Source: CAD feature listing. Evaluate the final solid. Frame: model axes, mm. Give positions to 0.01 mm unless a question says otherwise; leave off trailing zeros. Loops run counter-clockwise (first coordinate to the right, second up) from the corner with the lowest first, then second, coordinate; pieces in that order, holes last. Notation, with made-up numbers: M 26,-5.5 L 72,-5.5 A22 ccw 72,9.5 Z; hole C 26.5,42.5 d6. An arc over 180 degrees is marked long. Write item = value, one per line.
from build123d import *

# Parameters (mm, degrees)
F0_R     = 18.669
F1_DEPTH = 3.302


# Not quite as in the source:
# - a length typed as a fraction of an inch, garbled in the dataset ("3 / 203.2 mm" for 3/8 in), is restored


with BuildPart() as f1:
    # F0 (on Top) → F1 (new body)
    with BuildSketch(Plane.XY):
        Circle(F0_R)
        Polygon((-5.6092465283, 3.2385000208), (-3.7394976935, 6.477), (0, 6.477), (3.7394976935, 6.477), (5.6092465069, 3.238500058), (7.4789953871, 0), (5.6092465631, -3.2384999606), (3.7394976935, -6.477), (0, -6.477), (-3.7394976935, -6.477), (-5.6092464752, -3.2385001127), (-7.4789953871, 0), align=None, mode=Mode.SUBTRACT)
        with BuildLine():
            Line((0, 6.477), (-3.7394976935, 6.477))
            Line((-3.7394976935, 6.477), (-5.6092465283, 3.2385000208))
            ThreePointArc((-5.6092465283, 3.2385000208), (-3.2384999896, 5.6092465463), (0, 6.477))
        make_face()
        with BuildLine():
            Line((3.7394976935, 6.477), (0, 6.477))
            ThreePointArc((0, 6.477), (3.238499971, 5.609246557), (5.6092465069, 3.238500058))
            Line((5.6092465069, 3.238500058), (3.7394976935, 6.477))
        make_face()
        with BuildLine():
            ThreePointArc((5.6092465631, -3.2384999606), (3.2385000197, -5.6092465289), (0, -6.477))
            Line((0, -6.477), (3.7394976935, -6.477))
            Line((3.7394976935, -6.477), (5.6092465631, -3.2384999606))
        make_face()
        with BuildLine():
            Line((7.4789953871, 0), (5.6092465069, 3.238500058))
            ThreePointArc((5.6092465069, 3.238500058), (6.2563015682, 1.6763709874), (6.477, 0))
            ThreePointArc((6.477, 0), (6.2563015828, -1.6763709332), (5.6092465631, -3.2384999606))
            Line((5.6092465631, -3.2384999606), (7.4789953871, 0))
        make_face()
        with BuildLine():
            ThreePointArc((0, -6.477), (-3.2384999437, -5.6092465728), (-5.6092464752, -3.2385001127))
            Line((-5.6092464752, -3.2385001127), (-3.7394976935, -6.477))
            Line((-3.7394976935, -6.477), (0, -6.477))
        make_face()
        with BuildLine():
            ThreePointArc((-5.6092464752, -3.2385001127), (-6.477, -5.31e-08), (-5.6092465283, 3.2385000208))
            Line((-5.6092465283, 3.2385000208), (-7.4789953871, 0))
            Line((-7.4789953871, 0), (-5.6092464752, -3.2385001127))
        make_face()
    extrude(amount=F1_DEPTH)


solid = f1.part
1. Cut plane C-C, the plane x = 8.5. Return the cut outline in (y, z), then the cut area to 3 significant figures.
Derived:
outline = M -16.62,0 L 16.62,0 L 16.62,3.3 L -16.62,3.3 Z
area = 110 mm²
2. Cut plane A-A, the plane z = 0.7. Return the cut outline in (x, y).
Derived:
outline = C 0,0 d37.34; hole C 0,0 d12.95
3. Cut plane B-B, the plane y = -16. Return the cut outline in (x, z).
Derived:
outline = M -9.62,0 L 9.62,0 L 9.62,3.3 L -9.62,3.3 Z
4. Material intervals for probe 1 along Y at (x, z) = (5, 1.65); probe 2 along X at (y, z) = (1, 2.65); probe 3 along Y at (x, z) = (-3, 0.3), sorted ascending. Write a range as from..to.
Derived:
probe_1 = -17.99..-4.12, 4.12..17.99
probe_2 = -18.64..-6.4, 6.4..18.64
probe_3 = -18.43..-5.74, 5.74..18.43
